```python
from build123d import *

# Parameters (mm, degrees)
SKETCH_1_R          = 2.5
EXTRUDE_1_DEPTH     = 2
SKETCH_2_R          = 2.1
EXTRUDE_2_DEPTH     = 2
SKETCH_3_R          = 2.5
EXTRUDE_3_DEPTH     = 3.4
SKETCH_4_R          = 1.6
CUT_EXTRUDE_1_DEPTH = 9.201219422
FILLET_1_R          = 1


with BuildPart() as part:
    # Эскиз1 → Бобышка-Вытянуть1 (new body)
    with BuildSketch(Plane.XY):
        Circle(SKETCH_1_R)
    extrude(amount=EXTRUDE_1_DEPTH)

    # Эскиз2 → Бобышка-Вытянуть2 (add)
    with BuildSketch(Plane.XY.offset(2)):
        Circle(SKETCH_2_R)
    extrude(amount=EXTRUDE_2_DEPTH)

    # Эскиз3 → Бобышка-Вытянуть3 (add)
    with BuildSketch(Plane.XY.offset(4)):
        Circle(SKETCH_3_R)
    extrude(amount=EXTRUDE_3_DEPTH)

    # Эскиз4 → Вырез-Вытянуть1 (cut, through all)
    with BuildSketch(Plane.XY.offset(7.4)):
        Circle(SKETCH_4_R)
    extrude(amount=-CUT_EXTRUDE_1_DEPTH, mode=Mode.SUBTRACT)

    # Скругление1
    # the kernel refuses this fillet: 1 mm, written as the material it adds along each edge
    with BuildSketch(Plane(origin=(0, 0, 2), x_dir=(1, 0, 0), z_dir=(0, -1, 0))) as fillet_1_piece_1:
        with BuildLine():
            CenterArc((3.1, 0.8), FILLET_1_R, 180, 53.130102354)
            Line((2.5, 0), (2.488, -0.016))
            ThreePointArc((2.488, -0.016), (2.3, -0.02), (2.1, -0.02))
            Line((2.1, -0.02), (2.08, 0))
            Line((2.08, 0), (2.08, 0.8))
            Line((2.08, 0.8), (2.1, 0.8))
        make_face()
    revolve(axis=Axis((0, 0, 2), (0, 0, 1)))
    with BuildSketch(Plane(origin=(0, 0, 4), x_dir=(1, 0, 0), z_dir=(0, -1, 0))) as fillet_1_piece_2:
        with BuildLine():
            CenterArc((3.1, -0.8), FILLET_1_R, 126.869897646, 53.130102354)
            Line((2.1, -0.8), (2.08, -0.8))
            Line((2.08, -0.8), (2.08, 0))
            Line((2.08, 0), (2.1, 0.02))
            ThreePointArc((2.1, 0.02), (2.3, 0.02), (2.488, 0.016))
            Line((2.488, 0.016), (2.5, 0))
        make_face()
    revolve(axis=Axis((0, 0, 4), (0, 0, 1)))


solid = part.part
```
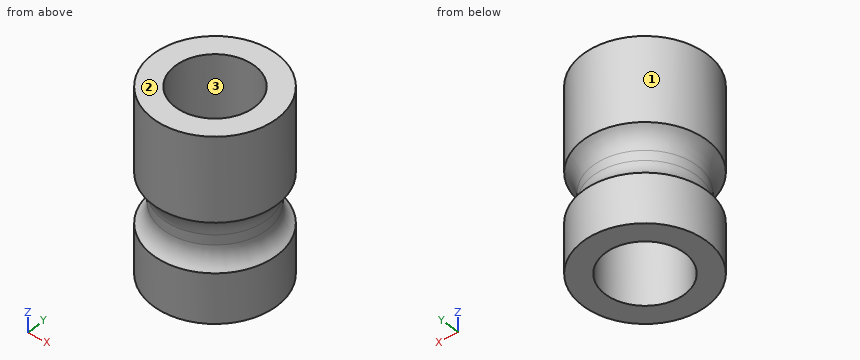
Could you check a few things on this model? Use its own coordinates, in mm. Face numbers are marked on the shaded views. Round coordinates to 2 decimals unless told otherwise and drop trailing zeros. Loops run counter-clockwise (first coordinate to the right, second up) from the corner with the lowest first, then second, coordinate; pieces in that order, holes last. Notation, with made-up numbers: (7.25, 1.25) -> (13.25, 1.25) arc R28 ccw to (13.25, 38.25) -> close; hole circle Ø2 at (74.5, -17). An arc over 180 degrees is marked (long way). One line per question, with ' | ' between items.
(1) Thinking about a two-plate mould opening in Y: for the marked faces 1, 2 and 3, which applies, released by +Y, released by -Y, zero draft, split by the parting line, or undercut?
Model answer:
face 1: split by the parting line | face 2: zero draft | face 3: undercut
(2) If we section it at C-C on z = 1: List the corners of the cut face in (x, y) for me.
Model answer:
outline: circle Ø5 at (0, 0); hole circle Ø3.2 at (0, 0)
(3) If we section it at A-A on y = 0: List the corners of the cut face in (x, z) for me, and give its area (3 significant figures).
Model answer:
outline: (-2.5, 0) -> (-1.6, 0) -> (-1.6, 7.4) -> (-2.5, 7.4) -> (-2.5, 4) arc R1 cw to (-2.1, 3.2) -> (-2.1, 2.8) arc R1 cw to (-2.5, 2) -> close; (1.6, 0) -> (2.5, 0) -> (2.5, 2) arc R1 cw to (2.1, 2.8) -> (2.1, 3.2) arc R1 cw to (2.5, 4) -> (2.5, 7.4) -> (1.6, 7.4) -> close | area: 12.1 mm^2
(4) If I drill on probe 1 along Y at (x, z) = (0, 5.5); probe 2 along Y at (x, z) = (0, 3.25); probe 3 along X at (y, z) = (-1, 2.5), over which ranges is the centre line in solid material (lowest first)?
Model answer:
probe 1: y = -2.5 to -1.6, 1.6 to 2.5 | probe 2: y = -2.1 to -1.6, 1.6 to 2.1 | probe 3: x = -1.9 to -1.25, 1.25 to 1.9
